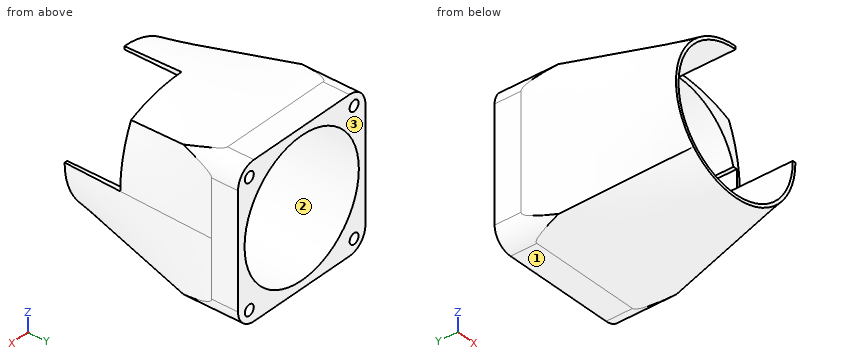
from build123d import *

# Parameters (mm, degrees)
F0_W      = 40
F0_H      = 40
F1_DEPTH  = 7
F3_R      = 18.75
F1_FACE_W = 40
F1_FACE_H = 40
F5_R      = 17.95
F6_DEPTH  = 47
F7_R      = 1.4
F8_DEPTH  = 7
F9_R      = 5
F11_DEPTH = 20
F13_DEPTH = 5


with BuildPart() as f1:
    # F0 (on Front) → F1 (new body)
    with BuildSketch(Plane.XZ):
        Rectangle(F0_W, F0_H)
    extrude(amount=F1_DEPTH)

    # F3 (on offset) → F4 section 0
    with BuildSketch(Plane.XZ.offset(47)):
        Circle(F3_R)
    # F1_face (on face) → F4 section 1
    with BuildSketch(Plane.XZ.offset(7)):
        Rectangle(F1_FACE_W, F1_FACE_H)
    loft()

    # F5 (on face) → F6 (cut, through all)
    with BuildSketch(Plane.XZ.offset(47)):
        Circle(F5_R)
    extrude(amount=-F6_DEPTH, mode=Mode.SUBTRACT)

    # F7 (on face) → F8 (cut, through all)
    with BuildSketch(Plane(origin=(0, 0, 0), x_dir=(-1, 0, 0), z_dir=(0, 1, 0))):
        with Locations((-16.45, 16.45)):
            Circle(F7_R)
        with Locations((16.45, 16.45)):
            Circle(F7_R)
        with Locations((-16.45, -16.45)):
            Circle(F7_R)
        with Locations((16.45, -16.45)):
            Circle(F7_R)
    extrude(amount=-F8_DEPTH, mode=Mode.SUBTRACT)

    # F9
    f9_edges = [f1.edges().sort_by_distance(p)[0] for p in [
        (20, -3.5, -20),
        (20, -3.5, 20),
        (-20, -3.5, 20),
        (-20, -3.5, -20),
    ]]
    fillet(f9_edges, radius=F9_R)

    # F10 (on face) → F11 (cut)
    with BuildSketch(Plane.XY.offset(20)):
        Polygon((0, -31.8655073643), (0, -47.008369118), (0, -48.6102327704), (19.3509273231, -48.6102327704), (19.3509273231, -31.8655073643), align=None)
    extrude(amount=-F11_DEPTH, mode=Mode.SUBTRACT)

    # F12 (on face) → F13 (cut)
    with BuildSketch(Plane.XZ.offset(31.8655073643)):
        with BuildLine():
            Line((15.9311909229, 0), (17.95, 0))
            ThreePointArc((17.95, 0), (17.7714847113, 2.5252388315), (17.2394895648, 5.0002499484))
            Line((17.2394895648, 5.0002499484), (15.9311909229, 5.0002499484))
            Line((15.9311909229, 5.0002499484), (15.9311909229, 0))
        make_face()
        with BuildLine():
            ThreePointArc((17.2394895648, 5.0002499484), (17.7714847113, 2.5252388315), (17.95, 0))
            Line((17.95, 0), (18.3052159846, 0))
            Line((18.3052159846, 0), (18.3052159846, 5.0002499484))
            Line((18.3052159846, 5.0002499484), (17.2394895648, 5.0002499484))
        make_face()
    extrude(amount=-F13_DEPTH, mode=Mode.SUBTRACT)


solid = f1.part
Work out the finished part from the listing and answer in its coordinate system (mm). Face numbers are marked on the shaded views. Give positions to 0.01 mm unless a question says otherwise; leave off trailing zeros. Answer as a JSON object with one key per item and string values. Group by question number.
1. Flat-ended cylindrical pins translate along their axes: pin 1 Ø4 at (x, y) = (-5, -42) entering from +Z; pin 2 Ø1.4 at (x, z) = (17, 16.5) entering from +Y; pin 3 Ø5 at (y, z) = (-31.5, -11) entering from +X; pin 4 Ø3.5 at (x, z) = (-16.45, 16.45) entering from +Y. Find the tip coordinate at first contact, or state that the pin passes through.
2. The mould has two halves that part along Z. Classify the marked faces 1, 2 and 3: released by +Z, released by -Z, zero draft, split by the parting line, or undercut.
3. Consider line 1 along Z through (x, y) = (-16.45, -2.75); line 2 along X through (y, z) = (-2, 16). Determine where each line is inside the solid, lowest interval first. Write a range as [from, to].
Result sheet:
{
 "1": {"pin 1": "stops at z = 18.73", "pin 2": "stops at y = -7", "pin 3": "stops at x = 18.35", "pin 4": "stops at y = 0"},
 "2": {"face 1": "released by -Z", "face 2": "undercut", "face 3": "zero draft"},
 "3": {"line 1": "z = [-19.79, -17.85], [-15.05, -7.18], [7.18, 15.05], [17.85, 19.79]", "line 2": "x = [-19.9, -17.78], [-15.12, -8.14], [8.14, 15.12], [17.78, 19.9]"}
}
